Geometry check sheet. Reference: the model listing, model coordinates, mm. Give positions to 0.01 mm unless a question says otherwise; leave off trailing zeros. Order: outer loops, then holes, each group sorted by start corner. A loop starts at its lowest first (then second) coordinate and runs counter-clockwise, first axis right, second up. Notation, with made-up numbers: M 89,6 L 141,6 A7 ccw 141,10 Z; hole C 22,-13 d10. An arc over 180 degrees is marked long. Use CSV: the item, a comma, the result in double quotes. Start each with the question number.
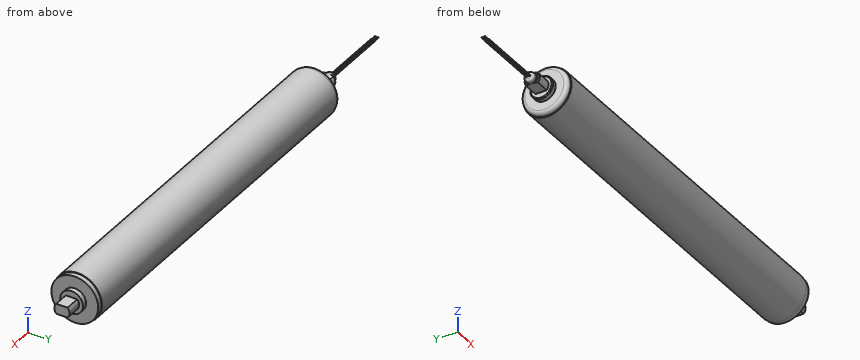
from build123d import *

# Parameters (mm, degrees)
CUT_EXTRUDE1_DEPTH = 326.112288294
CUT_EXTRUDE2_DEPTH = 322.126143439
LPATTERN1_COUNT    = 3
LPATTERN1_PITCH    = 1.25


with BuildPart() as part:
    # Sketch2 → Revolve2 (revolve)
    with BuildSketch(Plane.XY, mode=Mode.PRIVATE) as revolve2_sk:
        with BuildLine():
            Line((-4, 18.5), (0, 18.5))
            Line((0, 18.5), (0, 9))
            Line((0, 9), (4, 9))
            Line((4, 9), (4, 6))
            Line((4, 6), (16, 6))
            Line((16, 6), (16, 0))
            Line((16, 0), (-320, 0))
            Line((-320, 0), (-320, 2))
            ThreePointArc((-320, 2), (-319.414213562, 3.414213562), (-318, 4))
            Line((-318, 4), (-316, 4))
            Line((-316, 4), (-316, 5))
            Line((-316, 5), (-315, 6))
            Line((-315, 6), (-304, 6))
            Line((-304, 6), (-304, 8.2))
            Line((-304, 8.2), (-303.2, 9))
            Line((-303.2, 9), (-300, 9))
            Line((-300, 9), (-300, 15.5))
            ThreePointArc((-300, 15.5), (-299.121320344, 17.621320344), (-297, 18.5))
            Line((-297, 18.5), (-296, 18.5))
            Line((-296, 18.5), (-296, 19))
            Line((-296, 19), (-4, 19))
            Line((-4, 19), (-4, 18.5))
        make_face()
    revolve(revolve2_sk.sketch.rotate(Axis((-320, 0, 0), (1, 0, 0)), 180), axis=Axis((-320, 0, 0), (1, 0, 0)))

    # Sketch3 → Cut-Extrude1 (cut, through all)
    with BuildSketch(Plane(origin=(4, 0, 0), x_dir=(0, 0, -1), z_dir=(1, 0, 0))):
        with BuildLine():
            Line((-4, 4.472135955), (-4, -4.472135955))
            ThreePointArc((-4, -4.472135955), (-6, 0), (-4, 4.472135955))
        make_face()
        with BuildLine():
            Line((4, 4.472135955), (4, -4.472135955))
            ThreePointArc((4, -4.472135955), (6, 0), (4, 4.472135955))
        make_face()
    extrude(amount=CUT_EXTRUDE1_DEPTH, mode=Mode.SUBTRACT)

    # Sketch4 → Cut-Extrude2 (cut, through all)
    with BuildSketch(Plane(origin=(-304, 0, 0), x_dir=(0, 0, -1), z_dir=(1, 0, 0))):
        with BuildLine():
            Line((-4, 4.472135955), (-4, -4.472135955))
            ThreePointArc((-4, -4.472135955), (-6, 0), (-4, 4.472135955))
        make_face()
        with BuildLine():
            Line((4, 4.472135955), (4, -4.472135955))
            ThreePointArc((4, -4.472135955), (6, 0), (4, 4.472135955))
        make_face()
    extrude(amount=-CUT_EXTRUDE2_DEPTH, mode=Mode.SUBTRACT)

    # Sketch8 → Revolve3 (revolve)
    with BuildSketch(Plane.XY, mode=Mode.PRIVATE) as revolve3_sk:
        Polygon((-316, 1.75), (-371, 1.75), (-371, 1.5), (-376, 1.5), (-376, 1.25), (-316, 1.25), align=None)
    revolve3 = revolve(revolve3_sk.sketch.rotate(Axis((-377.615440864, 1.25, 0), (1, 0, 0)), 90), axis=Axis((-377.615440864, 1.25, 0), (1, 0, 0)))

    # LPattern1: Revolve3 ×3
    with Locations(*[(0, -i * LPATTERN1_PITCH, 0) for i in range(1, LPATTERN1_COUNT)]):
        add(revolve3)


solid = part.part
(1) Sectioned sample at B-B on x = -280. Record the cut outline in (y, z), then the cut area to 3 significant figures.
(2) Sectioned sample at A-A on x = -336. Record the cut outline in (y, z), then the cut area to 3 significant figures.
(3) Go/stop test with flat-tipped pins: P1, Ø10, axis at x = -77.5, z = -2, coming from the +Y side; P2, Ø1.5, axis at x = -257, y = 3, coming from the -Z side; P3, Ø10, axis at x = 10.5, y = -0.5, coming from the +Z side; P4, Ø2, axis at y = 11.5, z = 10.5, coming from the -X side. Record where each tip stops, or that it passes through.
(4) Thickness scan on line 1 (X direction, y = 12.5, z = -5); line 2 (Y direction, x = -275.5, z = -11); line 3 (Z direction, x = -263.5, y = -1.5). Record the ranges inside material, lowest first.
Responses:
1,outline,"C 0,0 d38"
1,area,"1,130 mm2"
2,outline,"C -1.25,0 d1; C 0,0 d1; C 1.25,0 d1"
2,area,"2.36 mm2"
3,P1,"y = 19"
3,P2,"z = -18.87"
3,P3,"z = 4"
3,P4,"x = -300"
4,line 1,"-300 to 0"
4,line 2,"-15.49 to 15.49"
4,line 3,"-18.94 to 18.94"
